Check sheet for the modelled part. Datum: model origin and axes. Units: mm. A direction names the side the tool comes from. Coordinates: 2 decimals unless noted, no trailing zeros. Write each loop counter-clockwise with the first axis right and the second up, starting at its lowest first coordinate (ties: lowest second). Pieces come first, ordered by that corner, then holes. Notation, with made-up numbers: M -2,0.25 L 11,0.25 A23 ccw 11,21.25 Z; hole C -24,-5.75 d3. An arc over 180 degrees is marked long. Answer as CSV lines item,"result". Start each with the question number.
1) Section check C-C (y = 6.5). Record the cut outline in (x, z), and give its area (3 significant figures).
2) Access from +Z, -Z, +X, -X, +Y, -Y to the whole of each face (thin tool, end or side, straight path). Record for faces 4 (the flat face through (0, 7, 19)), 5 (the cylindrical face through (-20.358, 43.727, 4.437)).
3) Draft check along Y on faces 1 (the cylindrical face through (-0.358, 43.727, 4.563)), 2 (the flat face through (0, 20, 20)), 3 (the flat face through (0, 5, 51)). Enter one of: +Y half, -Y half, draft (parallel to the pull), parting line (faces both ways), or undercut.
4) Section check A-A (y = 41). Record the cut outline in (x, z), and give its area (4 significant figures).
5) Material ranges on L1, parallel to Y at x = -8, z = 10.5; L2, parallel to Y at x = 5, z = 12; L3, parallel to Y at x = 20, z = 3, recorded low to high. Write a range as [from, to].
6) Go/stop test with flat-tipped pins: pin 1 Ø8 at (x, z) = (9.5, 12.5) entering from +Y; pin 2 Ø4 at (y, z) = (24, 19.5) entering from +X; pin 3 Ø7 at (x, y) = (20, 41) entering from +Z; pin 4 Ø2 at (x, y) = (-8, 21.5) entering from +Z. Record where each tip stops, or that it passes through.
from build123d import *

# Parameters (mm, degrees)
BOSS_EXTRUDE1_DEPTH      = 24
BOSS_EXTRUDE1_DEPTH_BACK = 24
SKETCH2_R                = 2.75
CUT_EXTRUDE1_DEPTH       = 9
SKETCH3_R                = 2.75
CUT_EXTRUDE2_DEPTH       = 9
SKETCH4_R                = 2.75
CUT_EXTRUDE3_DEPTH       = 9
SKETCH5_R                = 2.75
CUT_EXTRUDE4_DEPTH       = 9
SKETCH6_R                = 2.75
CUT_EXTRUDE5_DEPTH       = 10
SKETCH7_R                = 2.75
CUT_EXTRUDE6_DEPTH       = 10


with BuildPart() as part:
    # Sketch1 → Boss-Extrude1 (new body, two sides)
    with BuildSketch(Plane(origin=(0, 0, 0), x_dir=(0, 0, -1), z_dir=(1, 0, 0))) as boss_extrude1_sk:
        with BuildLine():
            Line((-50, 0), (-1, 0))
            ThreePointArc((-1, 0), (-0.292893219, 0.292893219), (0, 1))
            Line((0, 1), (0, 50))
            ThreePointArc((0, 50), (-0.292893219, 50.707106781), (-1, 51))
            Line((-1, 51), (-8, 51))
            ThreePointArc((-8, 51), (-8.707106781, 50.707106781), (-9, 50))
            Line((-9, 50), (-9, 31))
            Line((-9, 31), (-31, 9))
            Line((-31, 9), (-50, 9))
            ThreePointArc((-50, 9), (-50.707106781, 8.707106781), (-51, 8))
            Line((-51, 8), (-51, 1))
            ThreePointArc((-51, 1), (-50.707106781, 0.292893219), (-50, 0))
        make_face()
        with BuildLine():
            Line((-25.721825407, 5), (-20.999285733, 5))
            Line((-20.999285733, 5), (-16.494036438, 9.505249294))
            ThreePointArc((-16.494036438, 9.505249294), (-16.226979866, 9.987090789), (-16.255625497, 10.537245192))
            ThreePointArc((-16.255625497, 10.537245192), (-16.488859314, 11.683547702), (-16.418755424, 12.851234691))
            ThreePointArc((-16.418755424, 12.851234691), (-16.283360667, 13.048766752), (-16.046526031, 13.084263382))
            Line((-16.046526031, 13.084263382), (-14.300039569, 12.616293745))
            ThreePointArc((-14.300039569, 12.616293745), (-14.127781033, 12.492491496), (-14.080474622, 12.285701498))
            ThreePointArc((-14.080474622, 12.285701498), (-10.515075745, 10.515075774), (-12.285701539, 14.080474617))
            ThreePointArc((-12.285701539, 14.080474617), (-12.492491514, 14.127781045), (-12.616293745, 14.300039569))
            Line((-12.616293745, 14.300039569), (-13.084263382, 16.046526031))
            ThreePointArc((-13.084263382, 16.046526031), (-13.048766728, 16.283360705), (-12.851234602, 16.418755442))
            ThreePointArc((-12.851234602, 16.418755442), (-11.683774102, 16.488875269), (-10.537674556, 16.255773055))
            ThreePointArc((-10.537674556, 16.255773055), (-9.987311976, 16.226928716), (-9.505249294, 16.494036438))
            Line((-9.505249294, 16.494036438), (-5, 20.999285733))
            Line((-5, 20.999285733), (-5, 25.721825407))
            ThreePointArc((-5, 25.721825407), (-5.925974851, 27.107644706), (-7.560660172, 26.782485579))
            Line((-7.560660172, 26.782485579), (-26.782485579, 7.560660172))
            ThreePointArc((-26.782485579, 7.560660172), (-27.107644706, 5.925974851), (-25.721825407, 5))
        make_face(mode=Mode.SUBTRACT)
    extrude(amount=BOSS_EXTRUDE1_DEPTH)
    extrude(boss_extrude1_sk.sketch, amount=-BOSS_EXTRUDE1_DEPTH_BACK)

    # Sketch2 → Cut-Extrude1 (cut)
    with BuildSketch(Plane(origin=(0, 0, 0), x_dir=(-1, 0, 0), z_dir=(0, 1, 0))):
        with Locations((20, 41)):
            Circle(SKETCH2_R)
    extrude(amount=CUT_EXTRUDE1_DEPTH, mode=Mode.SUBTRACT)

    # Sketch3 → Cut-Extrude2 (cut)
    with BuildSketch(Plane(origin=(0, 0, 0), x_dir=(-1, 0, 0), z_dir=(0, 1, 0))):
        with Locations((-20, 41)):
            Circle(SKETCH3_R)
    extrude(amount=CUT_EXTRUDE2_DEPTH, mode=Mode.SUBTRACT)

    # Sketch4 → Cut-Extrude3 (cut)
    with BuildSketch(Plane.XY):
        with Locations((-20, 41)):
            Circle(SKETCH4_R)
    extrude(amount=CUT_EXTRUDE3_DEPTH, mode=Mode.SUBTRACT)

    # Sketch5 → Cut-Extrude4 (cut)
    with BuildSketch(Plane.XY):
        with Locations((20, 41)):
            Circle(SKETCH5_R)
    extrude(amount=CUT_EXTRUDE4_DEPTH, mode=Mode.SUBTRACT)

    # Sketch6 → Cut-Extrude5 (cut)
    with BuildSketch(Plane(origin=(0, 9, 0), x_dir=(1, 0, 0), z_dir=(0, 1, 0))):
        with Locations((0, -41)):
            Circle(SKETCH6_R)
    extrude(amount=-CUT_EXTRUDE5_DEPTH, mode=Mode.SUBTRACT)

    # Sketch7 → Cut-Extrude6 (cut)
    with BuildSketch(Plane.XY.offset(9)):
        with Locations((0, 41)):
            Circle(SKETCH7_R)
    extrude(amount=-CUT_EXTRUDE6_DEPTH, mode=Mode.SUBTRACT)


solid = part.part
Results found:
1,outline,"M -24,0 L 24,0 L 24,19.5 L -24,19.5 Z; M -24,27.22 L 24,27.22 L 24,51 L -24,51 Z; hole C -20,41 d5.5; hole C 0,41 d5.5; hole C 20,41 d5.5"
1,area,"2,010 mm2"
2,face 4,"+X, -X"
2,face 5,"+Z, -Z"
3,face 1,"undercut"
3,face 2,"+Y half"
3,face 3,"draft"
4,outline,"M -24,0 L -22.75,0 L -22.75,9 L -24,9 Z; M -17.25,0 L -2.75,0 L -2.75,9 L -17.25,9 Z; M 2.75,0 L 17.25,0 L 17.25,9 L 2.75,9 Z; M 22.75,0 L 24,0 L 24,9 L 22.75,9 Z"
4,area,"283.5 mm2"
5,L1,"y = [0, 10.53], [13.47, 16.24], [23.84, 29.5]"
5,L2,"y = [0, 9.9], [14.1, 16.5], [22.34, 28]"
5,L3,"y = [0, 38.25], [43.75, 51]"
6,pin 1,"stops at y = 50.87"
6,pin 2,"passes through"
6,pin 3,"stops at z = 9"
6,pin 4,"stops at z = 19.5"
